Could you check a few things on this model? Use its own coordinates, in mm. A direction names the side the tool comes from. Round coordinates to 2 decimals unless told otherwise and drop trailing zeros. Write each loop counter-clockwise with the first axis right and the second up, starting at its lowest first coordinate (ties: lowest second). Pieces come first, ordered by that corner, then holes. Notation, with made-up numbers: (66, 74) - (116, 74) arc R24 ccw to (116, 85) - close; hole circle Ø9 at (35, 63). An arc over 180 degrees is marked (long way). Put each result on its own line as item: value.
from build123d import *

# Parameters (mm, degrees)
SKETCH1_W               = 40
SKETCH1_H               = 8
BOSS_EXTRUDE1_DEPTH     = 60
SKETCH2_W               = 8
SKETCH2_H               = 20
BOSS_EXTRUDE2_DEPTH     = 30
CUT_EXTRUDE1_DEPTH      = 30
SKETCH6_R               = 1.5
CUT_EXTRUDE2_DEPTH      = 79.511145706
LPATTERN1_COUNT         = 4
LPATTERN1_PITCH         = 7
MIRROR3_COPY_1_SKETCH_R = 1.5
MIRROR3_COPY_1_DEPTH    = 79.511145706
MIRROR3_COPY_2_SKETCH_R = 1.5
MIRROR3_COPY_2_DEPTH    = 79.511145706
MIRROR3_COPY_3_SKETCH_R = 1.5
MIRROR3_COPY_3_DEPTH    = 79.511145706
SKETCH7_R               = 2
CUT_EXTRUDE3_DEPTH      = 30
SKETCH8_W               = 2
SKETCH8_H               = 60
BOSS_EXTRUDE3_DEPTH     = 2
FILLET1_R               = 1
FILLET1_OF_MIRROR4_R    = 1
FILLET2_R               = 0.5
FILLET3_R               = 5
SKETCH9_R               = 2
CUT_EXTRUDE4_DEPTH      = 10


# Some blends are built 0.0001 mm under size
with BuildPart() as part:
    # Sketch1 → Boss-Extrude1 (new body)
    with BuildSketch(Plane(origin=(0, 0, 0), x_dir=(1, 0, 0), z_dir=(0, 1, 0))):
        Rectangle(SKETCH1_W, SKETCH1_H)
    extrude(amount=-BOSS_EXTRUDE1_DEPTH)

    # Sketch2 → Boss-Extrude2 (add)
    with BuildSketch(Plane(origin=(20, 0, 0), x_dir=(0, 0, -1), z_dir=(1, 0, 0))):
        with Locations((0, -50)):
            Rectangle(SKETCH2_W, SKETCH2_H)
    boss_extrude2 = extrude(amount=BOSS_EXTRUDE2_DEPTH)

    # Sketch3 → Cut-Extrude1 (cut)
    with BuildSketch(Plane(origin=(50, 0, 0), x_dir=(0, 0, -1), z_dir=(1, 0, 0))):
        Polygon((1, -50), (1, -56), (4, -53), (4, -47), (1, -44), align=None)
    cut_extrude1 = extrude(amount=-CUT_EXTRUDE1_DEPTH, mode=Mode.SUBTRACT)

    # Sketch6 → Cut-Extrude2 (cut, through all)
    with BuildSketch(Plane.XY.offset(4)):
        with Locations((46.5, -50)):
            Circle(SKETCH6_R)
    cut_extrude2 = extrude(amount=-CUT_EXTRUDE2_DEPTH, mode=Mode.SUBTRACT)

    # LPattern1: Cut-Extrude2 ×4
    with Locations(*[(-i * LPATTERN1_PITCH, 0, 0) for i in range(1, LPATTERN1_COUNT)]):
        add(cut_extrude2, mode=Mode.SUBTRACT)

    # Mirror3: Boss-Extrude2, Cut-Extrude1, Cut-Extrude2 across plane
    add(boss_extrude2.mirror(Plane(origin=(0, 0, 0), x_dir=(0, 0, 1), z_dir=(1, 0, 0))))
    add(cut_extrude1.mirror(Plane(origin=(0, 0, 0), x_dir=(0, 0, 1), z_dir=(1, 0, 0))), mode=Mode.SUBTRACT)
    add(cut_extrude2.mirror(Plane(origin=(0, 0, 0), x_dir=(0, 0, 1), z_dir=(1, 0, 0))), mode=Mode.SUBTRACT)

    # Mirror3 copy 1 sketch → Mirror3 copy 1 (cut, through all)
    with BuildSketch(Plane(origin=(7, 0, 4), x_dir=(-1, 0, 0), z_dir=(0, 0, 1))):
        with Locations((46.5, 50)):
            Circle(MIRROR3_COPY_1_SKETCH_R)
    extrude(amount=-MIRROR3_COPY_1_DEPTH, mode=Mode.SUBTRACT)

    # Mirror3 copy 2 sketch → Mirror3 copy 2 (cut, through all)
    with BuildSketch(Plane(origin=(14, 0, 4), x_dir=(-1, 0, 0), z_dir=(0, 0, 1))):
        with Locations((46.5, 50)):
            Circle(MIRROR3_COPY_2_SKETCH_R)
    extrude(amount=-MIRROR3_COPY_2_DEPTH, mode=Mode.SUBTRACT)

    # Mirror3 copy 3 sketch → Mirror3 copy 3 (cut, through all)
    with BuildSketch(Plane(origin=(21, 0, 4), x_dir=(-1, 0, 0), z_dir=(0, 0, 1))):
        with Locations((46.5, 50)):
            Circle(MIRROR3_COPY_3_SKETCH_R)
    extrude(amount=-MIRROR3_COPY_3_DEPTH, mode=Mode.SUBTRACT)

    # Sketch7 → Cut-Extrude3 (cut)
    with BuildSketch(Plane.XY.offset(4)):
        with Locations((0, -30)):
            Circle(SKETCH7_R)
    extrude(amount=-CUT_EXTRUDE3_DEPTH, mode=Mode.SUBTRACT)

    # Sketch8 → Boss-Extrude3 (add)
    with BuildSketch(Plane(origin=(0, 0, -4), x_dir=(-1, 0, 0), z_dir=(0, 0, -1))):
        with Locations((-7.5, -30)):
            Rectangle(SKETCH8_W, SKETCH8_H)
    boss_extrude3 = extrude(amount=BOSS_EXTRUDE3_DEPTH)

    # Fillet1
    fillet1_edges = [part.edges().sort_by_distance(p)[0] for p in [
        (8.5, 0, -5),
        (6.5, 0, -5),
    ]]
    fillet(fillet1_edges, radius=FILLET1_R - 0.0001)  # a hair under: the kernel refuses the full size

    # Mirror4: Boss-Extrude3 across plane
    add(boss_extrude3.mirror(Plane(origin=(0, 0, 0), x_dir=(0, 0, 1), z_dir=(1, 0, 0))))

    # Fillet1 of Mirror4
    fillet1_of_mirror4_edges = [part.edges().sort_by_distance(p)[0] for p in [
        (-8.5, 0, -5),
        (-6.5, 0, -5),
    ]]
    fillet(fillet1_of_mirror4_edges, radius=FILLET1_OF_MIRROR4_R - 0.0001)  # a hair under: the kernel refuses the full size

    # Fillet2
    fillet2_edges = [part.edges().sort_by_distance(p)[0] for p in [
        (35, -44, -1),
        (35, -47, -4),
        (35, -53, -4),
        (35, -56, -1),
        (-35, -44, -1),
        (-35, -56, -1),
        (-35, -53, -4),
        (-35, -47, -4),
    ]]
    fillet(fillet2_edges, radius=FILLET2_R)

    # Fillet3
    # the kernel refuses this fillet: 5 mm, written as the material it adds along each edge
    with BuildSketch(Plane(origin=(20, -40, 4), x_dir=(1, 0, 0), z_dir=(0, 0, -1))) as fillet3_piece_1:
        with BuildLine():
            CenterArc((FILLET3_R, -FILLET3_R), FILLET3_R, 90, 90)
            Line((0, -FILLET3_R), (0, 0))
            Line((0, 0), (FILLET3_R, 0))
        make_face()
    extrude(amount=8)
    with BuildSketch(Plane(origin=(-20, -40, 4), x_dir=(-1, 0, 0), z_dir=(0, 0, -1))) as fillet3_piece_2:
        with BuildLine():
            CenterArc((FILLET3_R, FILLET3_R), FILLET3_R, 180, 90)
            Line((0, FILLET3_R), (0, 0))
            Line((0, 0), (FILLET3_R, 0))
        make_face()
    extrude(amount=8)
    # the kernel refuses this fillet: 5 mm, written as the material it takes off along each edge
    with BuildSketch(Plane(origin=(50, -60, -16.5), x_dir=(-1, 0, 0), z_dir=(0, 0, 1)), Plane(origin=(-50, -40, 16.5), x_dir=(0, -1, 0), z_dir=(0, 0, -1)), Plane(origin=(-50, -60, -16.5), x_dir=(0, 1, 0), z_dir=(0, 0, 1))) as fillet3_2_piece_1:
        with BuildLine():
            CenterArc((FILLET3_R, -FILLET3_R), FILLET3_R, 90, 90)
            Line((0, -FILLET3_R), (0, 0))
            Line((0, 0), (FILLET3_R, 0))
        make_face()
    extrude(amount=33, mode=Mode.SUBTRACT)
    with BuildSketch(Plane(origin=(50, -40, 16.5), x_dir=(0, -1, 0), z_dir=(0, 0, -1)), Plane(origin=(-20, 0, 16.5), x_dir=(1, 0, 0), z_dir=(0, 0, -1)), Plane(origin=(20, 0, -16.5), x_dir=(-1, 0, 0), z_dir=(0, 0, 1))) as fillet3_2_piece_2:
        with BuildLine():
            CenterArc((FILLET3_R, FILLET3_R), FILLET3_R, 180, 90)
            Line((0, FILLET3_R), (0, 0))
            Line((0, 0), (FILLET3_R, 0))
        make_face()
    extrude(amount=33, mode=Mode.SUBTRACT)

    # Sketch9 → Cut-Extrude4 (cut)
    with BuildSketch(Plane.XY.offset(4)):
        with Locations((0, -20)):
            Circle(SKETCH9_R)
    extrude(amount=-CUT_EXTRUDE4_DEPTH, mode=Mode.SUBTRACT)


solid = part.part
(1) Imagine slicing it at C-C, the plane z = 2. Give the number of separate pieces and of enclosed holes in the cut face, then the cut area to 3 significant figures.
Values found:
separate pieces: 1
enclosed holes: 10
area: 3,500 mm^2
(2) I'm going to push flat-ended pins straight in: pin 1 (2.5 mm diameter, centred on x = 25.5, y = -50, fed in from +Z); pin 2 (3 mm diameter, centred on x = -32.5, y = -49.5, fed in from -Z); pin 3 (3 mm diameter, centred on x = 21, z = -2.5, fed in from +Y); pin 4 (0.6 mm diameter, centred on y = -30, z = -5, fed in from +X). Where does each tip first touch, or does it pass through?
Values found:
pin 1: passes through
pin 2: stops at z = -1
pin 3: stops at y = -2.82
pin 4: stops at x = 8.5
(3) Imagine slicing it at A-A, the plane y = -20. List the corners of the cut face in (x, z) for me.
Values found:
outline: (-20, -4) - (-8.5, -4) - (-8.5, -6) - (-6.5, -6) - (-6.5, -4) - (-2, -4) - (-2, 4) - (-20, 4) - close; (2, -4) - (6.5, -4) - (6.5, -6) - (8.5, -6) - (8.5, -4) - (20, -4) - (20, 4) - (2, 4) - close
(4) Imagine slicing it at D-D, the plane x = 0. List the corners of the cut face in (y, z) for me, then the cut area to 3 significant figures.
Values found:
outline: (-60, -4) - (-32, -4) - (-32, 4) - (-60, 4) - close; (-28, -4) - (-22, -4) - (-22, 4) - (-28, 4) - close; (-18, -4) - (0, -4) - (0, 4) - (-18, 4) - close
area: 416 mm^2
(5) Imagine slicing it at B-B, the plane x = -39.5. List the corners of the cut face in (y, z) for me, then the cut area to 3 significant figures.
Values found:
outline: (-60, -4) - (-54.21, -4) arc R0.5 ccw to (-53.85, -3.15) - (-55.15, -1.85) arc R0.5 cw to (-54.79, -1) - (-51.5, -1) - (-51.5, 4) - (-60, 4) - close; (-48.5, -1) - (-45.21, -1) arc R0.5 cw to (-44.85, -1.85) - (-46.15, -3.15) arc R0.5 ccw to (-45.79, -4) - (-40, -4) - (-40, 4) - (-48.5, 4) - close
area: 118 mm^2
(6) If we mould it in two halves opening along Y, with no side actions, what happens to faces 4 (the face through (-25.175, -48.536, 1.535)), 5 (the face through (19, -2, 0)), 6 (the face through (50, -50, 2))? For each: pulls with the +Y half, pulls with the -Y half, needs draft (parallel to the pull), parting line crosses it, or undercut.
Values found:
face 4: undercut
face 5: pulls with the +Y half
face 6: needs draft
(7) For faces 1 (the face through (-20, -20, 0)), 2 (the face through (35, -40, 0)), 3 (the face through (-35, -50, -1)), which set-ups out of +Z, -Z, +X, -X, +Y, -Y let a thin tool reach every point of the face, with its end or its side?
Values found:
face 1: +Z, -Z, -X, +Y
face 2: +Z, -Z, +X, +Y
face 3: -X
(8) Please list where these lines run through material, in increasing order: probe 1 along Y at (x, z) = (0, -0.25); probe 2 along Y at (x, z) = (-39.5, 1.45); probe 3 along Y at (x, z) = (-28.5, -1.5). Write a range as from..to.
Values found:
probe 1: y = -60..-32, -28..-22, -18..0
probe 2: y = -60..-51.5, -48.5..-40
probe 3: y = -60..-55.29, -44.71..-40
